Source: CAD feature listing. Evaluate the final solid. Frame: model axes, mm. A direction names the side the tool comes from. Round coordinates to 2 decimals unless told otherwise and drop trailing zeros. Order: outer loops, then holes, each group sorted by start corner. A loop starts at its lowest first (then second) coordinate and runs counter-clockwise, first axis right, second up. Notation, with made-up numbers: (60, 59.25) -> (72, 59.25) arc R26 ccw to (72, 76.25) -> close; hole circle Ø6 at (15, -34.5). An arc over 180 degrees is marked (long way). One line per item, written item: value. Start each with the question number.
1) Pin query (flat end, axial travel): P1, Ø2, axis at x = 1, z = -13.5, coming from the -Y side; P2, Ø4, axis at x = 0, z = 0, coming from the +Y side; P3, Ø2, axis at x = -1, y = -0.5, coming from the -Z side. Return the tip coordinate at first contact, or that it passes through.
2) Reachability of faces 4 (the face through (1.04, 2.5, -1.3)), 5 (the face through (0.9, -1.52, -2.86)), 6 (the face through (3.5, 1.52, 20.07)) from +Z, -Z, +X, -X, +Y, -Y: full face, straight path, thin tool, end or side. Return the list, or none.
3) Section C-C (z = -12). Return the cut outline in (x, y).
4) Mould query, pull axis Z, two halves, no side actions, for faces 1 (the face through (0.03, 1.52, 12.25)), 2 (the face through (-1, 3, -13)), 3 (the face through (3.57, 1.52, -20)). Classes: pulls with the +Z half, pulls with the -Z half, needs draft (parallel to the pull), parting line crosses it, or undercut.
5) Ray query, L1, parallel to X at y = 1.7, z = 13; L2, parallel to X at y = 1.1, z = 0; L3, parallel to Y at x = -3.5, z = 5. Return the intervals inside material, ascending.
6) Section D-D (y = -1). Return the cut outline in (x, z), and give its area (3 significant figures).
7) Section A-A (z = 0). Return the cut outline in (x, y).
8) Section B-B (y = 1.2). State how many separate pieces and enclosed holes the cut face has, and give its area (3 significant figures).
```python
from build123d import *

# Parameters (mm, degrees)
SKETCH1_W           = 10
SKETCH1_H           = 43
BOSS_EXTRUDE1_DEPTH = 3
FILLET1_R           = 5
SKETCH2_R           = 4.5
BOSS_EXTRUDE2_DEPTH = 3
DRAFT1_ANGLE        = 10
SKETCH3_R           = 3
CUT_EXTRUDE1_DEPTH  = 3
SKETCH4_R           = 1.5
CUT_EXTRUDE2_DEPTH  = 23.27666941
SKETCH5_R           = 5.5
CUT_EXTRUDE3_DEPTH  = 0.5
FILLET2_R           = 0.5
SKETCH6_R           = 1.25
SKETCH6_R_2         = 0.75
CUT_EXTRUDE4_DEPTH  = 23.874658467


with BuildPart() as part:
    # Sketch1 → Boss-Extrude1 (new body)
    with BuildSketch(Plane(origin=(0, 0, 0), x_dir=(1, 0, 0), z_dir=(0, 1, 0))):
        Rectangle(SKETCH1_W, SKETCH1_H)
    extrude(amount=BOSS_EXTRUDE1_DEPTH)

    # Fillet1
    fillet1_edges = [part.edges().sort_by_distance(p)[0] for p in [
        (-5, 1.5, -21.5),
        (5, 1.5, -21.5),
        (5, 1.5, 21.5),
        (-5, 1.5, 21.5),
    ]]
    fillet(fillet1_edges, radius=FILLET1_R - 0.0001)  # a hair under: the kernel refuses the full size

    # Sketch2 → Boss-Extrude2 (add)
    with BuildSketch(Plane(origin=(0, 0, 0), x_dir=(1, 0, 0), z_dir=(0, 1, 0))):
        with Locations(Location((0, 0, 0), (0, 0, 270))):
            Circle(SKETCH2_R)
    extrude(amount=-BOSS_EXTRUDE2_DEPTH)

    # Draft1
    draft1_faces = [part.faces().sort_by_distance(p)[0] for p in [
        (0, -1.5, -4.5),
    ]]
    draft(draft1_faces, Plane(origin=(0, 0, 0), x_dir=(0, 0, -1), z_dir=(0, -1, 0)), DRAFT1_ANGLE)

    # Sketch3 → Cut-Extrude1 (cut)
    with BuildSketch(Plane.XZ.offset(3)):
        with Locations(Location((0, 0, 0), (0, 0, 270))):
            Circle(SKETCH3_R)
    extrude(amount=-CUT_EXTRUDE1_DEPTH, mode=Mode.SUBTRACT)

    # Sketch4 → Cut-Extrude2 (cut, through all)
    with BuildSketch(Plane.XZ):
        with Locations(Location((0, 0, 0), (0, 0, 270))):
            Circle(SKETCH4_R)
    extrude(amount=-CUT_EXTRUDE2_DEPTH, mode=Mode.SUBTRACT)

    # Sketch5 → Cut-Extrude3 (cut)
    with BuildSketch(Plane(origin=(0, 3, 0), x_dir=(1, 0, 0), z_dir=(0, 1, 0))):
        Circle(SKETCH5_R)
    extrude(amount=-CUT_EXTRUDE3_DEPTH, mode=Mode.SUBTRACT)

    # Fillet2
    fillet2_edges = [part.edges().sort_by_distance(p)[0] for p in [
        (-5, 2.75, -2.291287847),
        (5, 2.75, -2.291287847),
        (-5, 2.75, 2.291287847),
        (5, 2.75, 2.291287847),
    ]]
    fillet(fillet2_edges, radius=FILLET2_R)

    # Sketch6 → Cut-Extrude4 (cut, through all)
    with BuildSketch(Plane(origin=(0, 3, 0), x_dir=(1, 0, 0), z_dir=(0, 1, 0))):
        with Locations(Location((0, 12, 0), (0, 0, 270))):
            Circle(SKETCH6_R)
        with Locations(Location((0, 16, 0), (0, 0, 270))):
            Circle(SKETCH6_R_2)
        with Locations(Location((0, 8, 0), (0, 0, 270))):
            Circle(SKETCH6_R_2)
        with Locations(Location((0, -17, 0), (0, 0, 270))):
            Circle(SKETCH6_R)
        with Locations(Location((0, -9, 0), (0, 0, 270))):
            Circle(SKETCH6_R)
        with Locations(Location((0, -13, 0), (0, 0, 270))):
            Circle(SKETCH6_R_2)
    extrude(amount=-CUT_EXTRUDE4_DEPTH, mode=Mode.SUBTRACT)


solid = part.part
```
Findings:
1. P1: y = 0
1. P2: y = 2.5
1. P3: z = -21.5
2. face 4: +Y
2. face 5: -Y
2. face 6: +Z, +X, +Y, -Y
3. outline: (-5, 0) -> (-1.25, 0) -> (-1.25, 3) -> (-5, 3) -> close; (1.25, 0) -> (5, 0) -> (5, 3) -> (1.25, 3) -> close
4. face 1: undercut
4. face 2: needs draft
4. face 3: pulls with the -Z half
5. L1: -5 to -0.75, 0.75 to 5
5. L2: -5 to -1.5, 1.5 to 5
5. L3: 0 to 3
6. outline: circle Ø8.65 at (0, 0); hole circle Ø6 at (0, 0)
6. area: 30.5 mm2
7. outline: (-5, 0) -> (-4.5, 0) -> (-3.97, -3) -> (-3, -3) -> (-3, 0) -> (-1.5, 0) -> (-1.5, 2.5) -> (-5, 2.5) -> close; (1.5, 0) -> (3, 0) -> (3, -3) -> (3.97, -3) -> (4.5, 0) -> (5, 0) -> (5, 2.5) -> (1.5, 2.5) -> close
8. separate pieces: 1
8. enclosed holes: 7
8. area: 381 mm2
